Input: part model. Units: mm. Frame: model coordinates. A direction names the side the tool comes from. Round coordinates to 2 decimals unless told otherwise and drop trailing zeros. Order: outer loops, then holes, each group sorted by start corner. A loop starts at its lowest first (then second) coordinate and runs counter-clockwise, first axis right, second up. Notation, with made-up numbers: (-1, 39.25) -> (39, 39.25) arc R17 ccw to (39, 59.25) -> close; hole circle Ø4 at (25.5, -10). An arc over 180 degrees is marked (long way). Use a Markdown table: item, result.
from build123d import *

# Parameters (mm, degrees)
PAD002_DEPTH                  = 2
PAD003_DEPTH                  = 2
SKETCH005_R                   = 1.5
POCKET001_DEPTH               = 226.7018
SKETCH005_MIRRORED002_2_R     = 1.5
POCKET001_MIRRORED002_2_DEPTH = 226.7018
CHAMFER_SIZE                  = 2


with BuildPart() as part:
    # Sketch003 → Pad002 (new body)
    with BuildSketch(Plane.XY.offset(31)):
        with BuildLine():
            Line((-42, 15), (42, 15))
            ThreePointArc((46, 11), (44.828427, 13.828427), (42, 15))
            Line((46, 11), (46, -11))
            ThreePointArc((42, -15), (44.828427, -13.828427), (46, -11))
            Line((42, -15), (-42, -15))
            ThreePointArc((-46, -11), (-44.828427, -13.828427), (-42, -15))
            Line((-46, -11), (-46, 11))
            ThreePointArc((-42, 15), (-44.828427, 13.828427), (-46, 11))
        make_face()
    extrude(amount=PAD002_DEPTH)

    # Sketch004 → Pad003 (join)
    with BuildSketch(Plane.XY.offset(31)):
        with BuildLine():
            Line((-42, 13), (42, 13))
            ThreePointArc((44, 11), (43.414214, 12.414214), (42, 13))
            Line((44, 11), (44, -11))
            ThreePointArc((42, -13), (43.414214, -12.414214), (44, -11))
            Line((42, -13), (-42, -13))
            ThreePointArc((-44, -11), (-43.414214, -12.414214), (-42, -13))
            Line((-44, -11), (-44, 11))
            ThreePointArc((-42, 13), (-43.414214, 12.414214), (-44, 11))
        make_face()
    extrude(amount=-PAD003_DEPTH)

    # Sketch005 → Pocket001 (cut, through all)
    with BuildSketch(Plane.XY):
        with Locations((-42, 11)):
            Circle(SKETCH005_R)
    pocket001 = extrude(amount=POCKET001_DEPTH, mode=Mode.SUBTRACT)

    # Sketch005 Mirrored002 2 → Pocket001 Mirrored002 2 (cut, through all)
    with BuildSketch(Plane(origin=(0, 0, 0), x_dir=(-1, 0, 0), z_dir=(0, 0, -1))):
        with Locations((-42, 11)):
            Circle(SKETCH005_MIRRORED002_2_R)
    pocket001_mirrored002_2 = extrude(amount=-POCKET001_MIRRORED002_2_DEPTH, mode=Mode.SUBTRACT)

    # Mirrored003: Pocket001, Pocket001 Mirrored002 2 across Sketch005 H_Axis
    add(pocket001.mirror(Plane.ZX), mode=Mode.SUBTRACT)
    add(pocket001_mirrored002_2.mirror(Plane.ZX), mode=Mode.SUBTRACT)

    # Chamfer
    chamfer_edges = [part.edges().sort_by_distance(p)[0] for p in [
        (-43.5, -11, 33),
        (-43.5, 11, 33),
        (43.5, 11, 33),
        (43.5, -11, 33),
    ]]
    chamfer(chamfer_edges, length=CHAMFER_SIZE)


solid = part.part
1) Cut plane B-B on z = 29.75. Return loops of the section in (x, y).
Answer key:
| item | result |
|---|---|
| outline | (-44, -11) arc R2 ccw to (-42, -13) -> (42, -13) arc R2 ccw to (44, -11) -> (44, 11) arc R2 ccw to (42, 13) -> (-42, 13) arc R2 ccw to (-44, 11) -> close; hole circle Ø3 at (-42, -11); hole circle Ø3 at (-42, 11); hole circle Ø3 at (42, -11); hole circle Ø3 at (42, 11) |
2) Contact query for flat-ended pins moving along their axis: P1, Ø5, axis at x = 42, y = -11, coming from the -Z side; P2, Ø1, axis at x = -9.5, z = 30, coming from the +Y side; P3, Ø1.6, axis at x = -3.5, z = 29.5, coming from the -Y side; P4, Ø1, axis at y = 2.5, z = 30, coming from the +X side. Output: stop coordinate, or through.
Answer key:
| item | result |
|---|---|
| P1 | stops at z = 29 |
| P2 | stops at y = 13 |
| P3 | stops at y = -13 |
| P4 | stops at x = 44 |
3) Ray query, probe 1 along Y at (x, z) = (42, 30.05); probe 2 along Y at (x, z) = (-42, 31.6); probe 3 along X at (y, z) = (13, 32.35). Return the intervals inside material, ascending.
Answer key:
| item | result |
|---|---|
| probe 1 | y = -13 to -12.5, -9.5 to 9.5, 12.5 to 13 |
| probe 2 | y = -15 to -13.1, -8.9 to 8.9, 13.1 to 15 |
| probe 3 | x = -45.46 to -44.03, -39.97 to 39.97, 44.03 to 45.46 |
4) Set-up query: faces 1 (the face through (43.4, -12.43, 30.01)), 2 (the face through (-43.43, -12.4, 30.01)), 3 (the face through (44, 0, 30)). Return all of +Z, -Z, +X, -X, +Y, -Y with unobstructed straight access to the full face (end or side cutting, diameter ignored); none if empty.
Answer key:
| item | result |
|---|---|
| face 1 | -Z, +X, -Y |
| face 2 | -Z, -X, -Y |
| face 3 | -Z, +X, +Y, -Y |
5) Cut plane A-A on x = -8.5. Return loops of the section in (y, z).
Answer key:
| item | result |
|---|---|
| outline | (-15, 31) -> (-13, 31) -> (-13, 29) -> (13, 29) -> (13, 31) -> (15, 31) -> (15, 33) -> (-15, 33) -> close |
6) Cut plane C-C on y = -0.25. Return loops of the section in (x, z), and give its area (3 significant figures).
Answer key:
| item | result |
|---|---|
| outline | (-46, 31) -> (-44, 31) -> (-44, 29) -> (44, 29) -> (44, 31) -> (46, 31) -> (46, 33) -> (-46, 33) -> close |
| area | 360 mm^2 |
7) Draft query along Y for faces 4 (the face through (-43.5, 11.07, 29.99)), 5 (the face through (46, 0, 32)), 6 (the face through (-43.4, 12.43, 30.01)). Return one class per face: released by +Y, released by -Y, zero draft, split by the parting line, or undercut.
Answer key:
| item | result |
|---|---|
| face 4 | undercut |
| face 5 | zero draft |
| face 6 | released by +Y |
